CAD build for the part. Positions are in the model's coordinates, mm. Face numbers are marked on the shaded views. Give positions to 0.01 mm unless a question says otherwise; leave off trailing zeros. Order: outer loops, then holes, each group sorted by start corner. A loop starts at its lowest first (then second) coordinate and runs counter-clockwise, first axis right, second up.
from build123d import *

# Parameters (mm, degrees)
SKETCH_1_R          = 12.5
EXTRUDE_2_DEPTH     = 35
SKETCH_4_R          = 14.624451674
CUT_EXTRUDE_1_DEPTH = 15


with BuildPart() as part:
    # 스케치1 → 보스-돌출2 (new body)
    with BuildSketch(Plane.XY):
        Circle(SKETCH_1_R)
    extrude(amount=EXTRUDE_2_DEPTH)

    # 스케치3 → 컷-회전1 (revolve, cut)
    with BuildSketch(Plane(origin=(0, 0, 0), x_dir=(1, 0, 0), z_dir=(0, 1, 0))):
        with BuildLine():
            Line((0, -21), (0, -41))
            ThreePointArc((0, -41), (-10, -31), (0, -21))
        make_face()
    revolve(axis=Axis((0, 0, 35), (0, 0, -1)), mode=Mode.SUBTRACT)

    # 스케치4 → 컷-돌출1 (cut)
    with BuildSketch(Plane(origin=(0, 0, 0), x_dir=(-1, 0, 0), z_dir=(0, 0, -1))):
        Circle(SKETCH_4_R)
    extrude(amount=-CUT_EXTRUDE_1_DEPTH, mode=Mode.SUBTRACT)

    # 스케치5 → 컷-회전2 (revolve, cut)
    with BuildSketch(Plane(origin=(0, 0, 0), x_dir=(1, 0, 0), z_dir=(0, 1, 0))):
        with BuildLine():
            Line((0, -20.75), (0, -41.25))
            ThreePointArc((0, -41.25), (-10.25, -31), (0, -20.75))
        make_face()
    revolve(axis=Axis((0, 0, 35), (0, 0, -1)), mode=Mode.SUBTRACT)


solid = part.part
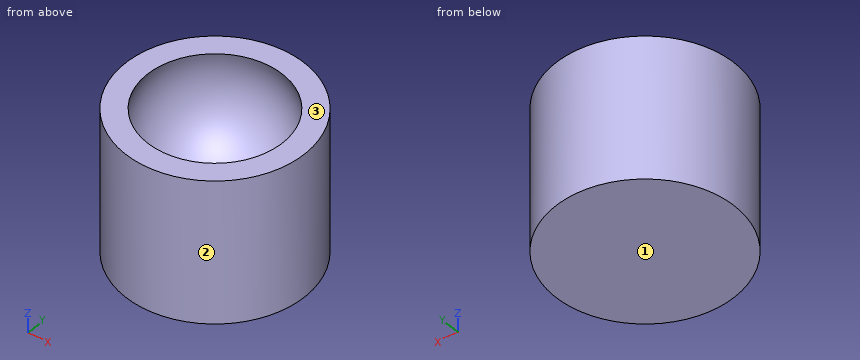
1. Saw through at A-A on x = 4.75. Give the cut face in (y, z), plus the area to 3 significant figures.
2. Pin check, flat tips, straight feed: P1, Ø4, axis at x = 1.5, y = 2, coming from the +Z side; P2, Ø4, axis at x = 7.5, z = 24, coming from the +Y side (3 decimals); P3, Ø4, axis at x = -5, z = 28.5, coming from the -Y side. Stop position of each tip, or through.
3. Saw through at D-D on z = 24.5. Give the cut face in (x, y), plus the area to 3 significant figures.
4. Wall check: line 1 (Y direction, x = 8.5, z = 33.25); line 2 (X direction, y = 1, z = 29); line 3 (Y direction, x = -5.5, z = 32). Give the ranges that are in metal, low to high.
5. Saw through at B-B on z = 19. Give the cut face in (x, y).
6. Mould opens along Z. For the marked faces 1, 2 and 3 say: released by +Z, released by -Z, zero draft, split by the parting line, or undercut.
7. Saw through at C-C on y = -1.25. Give the cut face in (x, z), plus the area to 3 significant figures.
Reported:
1. outline: (-11.56, 15) - (11.56, 15) - (11.56, 35) - (8.15, 35) arc R9.08 cw (long way) to (-8.15, 35) - (-11.56, 35) - close
1. area: 263 mm2
2. P1: stops at z = 21.79
2. P2: stops at y = 11.225
2. P3: stops at y = -12.13
3. outline: circle Ø25 at (0, 0); hole circle Ø15.85 at (0, 0)
3. area: 294 mm2
4. line 1: y = -9.17 to -5.27, 5.27 to 9.17
4. line 2: x = -12.46 to -10, 10 to 12.46
4. line 3: y = -11.22 to -8.59, 8.59 to 11.22
5. outline: circle Ø25 at (0, 0)
6. face 1: released by -Z
6. face 2: zero draft
6. face 3: released by +Z
7. outline: (-12.44, 15) - (12.44, 15) - (12.44, 35) - (9.35, 35) arc R10.17 cw (long way) to (-9.35, 35) - (-12.44, 35) - close
7. area: 256 mm2
